from build123d import *

# Parameters (mm, degrees)
SKETCH1_R           = 4
BOSS_EXTRUDE1_DEPTH = 15
CUT_EXTRUDE1_REACH  = 24
SKETCH2_R           = 2
FILLET1_R           = 0.25


with BuildPart() as part:
    # Sketch1 → Boss-Extrude1 (new body, symmetric)
    with BuildSketch(Plane.XY):
        Polygon((17, -11), (-17, -11), (-17, 7), (-8.3, 7), (-4, 11), (4, 11), (8.3, 7), (17, 7), align=None)
        Circle(SKETCH1_R, mode=Mode.SUBTRACT)
    extrude(amount=BOSS_EXTRUDE1_DEPTH, both=True)

    # Sketch2 → Cut-Extrude1 (cut, up to next)
    with BuildSketch(Plane.XZ.offset(11), mode=Mode.PRIVATE) as cut_extrude1_sk1:
        with Locations((12, 9)):
            Circle(SKETCH2_R)
    cut_extrude1_tool1 = extrude(cut_extrude1_sk1.sketch, amount=-CUT_EXTRUDE1_REACH, mode=Mode.PRIVATE) & part.part
    add(cut_extrude1_tool1.solids().sort_by_distance((12, -11, 9))[0], mode=Mode.SUBTRACT)
    # Sketch2 → Cut-Extrude1 (cut, up to next)
    with BuildSketch(Plane.XZ.offset(11), mode=Mode.PRIVATE) as cut_extrude1_sk2:
        with Locations((-12, 9)):
            Circle(SKETCH2_R)
    cut_extrude1_tool2 = extrude(cut_extrude1_sk2.sketch, amount=-CUT_EXTRUDE1_REACH, mode=Mode.PRIVATE) & part.part
    add(cut_extrude1_tool2.solids().sort_by_distance((-12, -11, 9))[0], mode=Mode.SUBTRACT)
    # Sketch2 → Cut-Extrude1 (cut, up to next)
    with BuildSketch(Plane.XZ.offset(11), mode=Mode.PRIVATE) as cut_extrude1_sk3:
        with Locations((12, -9)):
            Circle(SKETCH2_R)
    cut_extrude1_tool3 = extrude(cut_extrude1_sk3.sketch, amount=-CUT_EXTRUDE1_REACH, mode=Mode.PRIVATE) & part.part
    add(cut_extrude1_tool3.solids().sort_by_distance((12, -11, -9))[0], mode=Mode.SUBTRACT)
    # Sketch2 → Cut-Extrude1 (cut, up to next)
    with BuildSketch(Plane.XZ.offset(11), mode=Mode.PRIVATE) as cut_extrude1_sk4:
        with Locations((-12, -9)):
            Circle(SKETCH2_R)
    cut_extrude1_tool4 = extrude(cut_extrude1_sk4.sketch, amount=-CUT_EXTRUDE1_REACH, mode=Mode.PRIVATE) & part.part
    add(cut_extrude1_tool4.solids().sort_by_distance((-12, -11, -9))[0], mode=Mode.SUBTRACT)

    # Fillet1
    fillet1_edges = [part.edges().sort_by_distance(p)[0] for p in [
        (0, 11, -15),
        (6.15, 9, -15),
        (12.65, 7, -15),
        (17, -2, -15),
        (6.15, 9, 15),
        (17, -11, 0),
        (-17, -11, 0),
        (-17, 7, 0),
        (-8.3, 7, 0),
        (-4, 11, 0),
        (4, 11, 0),
        (8.3, 7, 0),
        (17, 7, 0),
        (0, 11, 15),
        (-6.15, 9, 15),
        (-12.65, 7, 15),
        (-17, -2, 15),
        (0, -11, 15),
        (17, -2, 15),
        (0, -11, -15),
        (12.65, 7, 15),
        (-17, -2, -15),
        (-12.65, 7, -15),
        (-6.15, 9, -15),
    ]]
    fillet(fillet1_edges, radius=FILLET1_R)


solid = part.part
The listing builds one solid part. Answer for the finished solid, in the listing's coordinates (mm). A direction names the side the tool comes from. Round coordinates to 2 decimals unless told otherwise and drop trailing zeros. Order: outer loops, then holes, each group sorted by start corner. A loop starts at its lowest first (then second) coordinate and runs counter-clockwise, first axis right, second up. Notation, with made-up numbers: (6.5, 39) - (32.5, 39) arc R21 cw to (32.5, 52) - close; hole circle Ø1 at (62.5, 48.25). An arc over 180 degrees is marked (long way). Write item = value, one per line. Start each with the question number.
1) Section D-D, the plane x = 0 is taken. Write down the section's boundary in (y, z), plus the area to 3 significant figures.
2) Given pin 1 (4.5 mm diameter, centred on x = -12, z = 9, fed in from +Y); pin 2 (6.5 mm diameter, centred on x = -11, z = -3.5, fed in from +Y); pin 3 (2.5 mm diameter, centred on x = 12, z = 9, fed in from -Y), each flat-ended and moving along its own axis, determine where each tip first touches the part or whether it passes through.
3) For faces 4 (the flat face through (13, 7, 0)), 5 (the cylindrical face through (10.526, -2.126, -7.648)), 6 (the flat face through (-13, 7, 0)), determine the directions among +Z, -Z, +X, -X, +Y, -Y from which every point of the face is accessible in a straight line to the end or side of a thin tool.
4) Section B-B, the plane y = 0 is taken. Write down the section's boundary in (x, z), plus the area to 3 significant figures.
5) For a pull along Y with two mould halves and no side action, classify faces 1 (the flat face through (0, -5, -15)), 2 (the cylindrical face through (-6.07, 8.97, 14.93)), 3 (the cylindrical face through (-0.867, -3.905, -0.21)) as released by +Y, released by -Y, zero draft, split by the parting line, or undercut.
6) Section C-C, the plane x = -12 is taken. Write down the section's boundary in (y, z), plus the area to 3 significant figures.
7) Section A-A, the plane z = -9 is taken. Write down the section's boundary in (x, y).
8) Straight lines are drawn through the part: L1, parallel to Z at x = -12, y = -3.25; L2, parallel to Y at x = 0, z = -7.5; L3, parallel to X at y = 2.75, z = 7.5. For each, find the intervals that lie inside material, in ascending order.
Results list:
q1.outline = (-11, -14.75) arc R0.25 ccw to (-10.75, -15) - (-4, -15) - (-4, 15) - (-10.75, 15) arc R0.25 ccw to (-11, 14.75) - close; (4, -15) - (10.75, -15) arc R0.25 ccw to (11, -14.75) - (11, 14.75) arc R0.25 ccw to (10.75, 15) - (4, 15) - close
q1.area = 420 mm^2
q2.pin_1 = 7
q2.pin_2 = 7.51
q2.pin_3 = through
q3.face_4 = +Z, -Z, +X, +Y
q3.face_5 = +Y, -Y
q3.face_6 = +Z, -Z, -X, +Y
q4.outline = (-17, -14.75) arc R0.25 ccw to (-16.75, -15) - (-4, -15) - (-4, 15) - (-16.75, 15) arc R0.25 ccw to (-17, 14.75) - close; (4, -15) - (16.75, -15) arc R0.25 ccw to (17, -14.75) - (17, 14.75) arc R0.25 ccw to (16.75, 15) - (4, 15) - close; hole circle Ø4 at (-12, -9); hole circle Ø4 at (-12, 9); hole circle Ø4 at (12, -9); hole circle Ø4 at (12, 9)
q4.area = 730 mm^2
q5.face_1 = zero draft
q5.face_2 = released by +Y
q5.face_3 = undercut
q6.outline = (-11, -14.75) arc R0.25 ccw to (-10.75, -15) - (6.75, -15) arc R0.25 ccw to (7, -14.75) - (7, -11) - (-11, -11) - close; (-11, -7) - (7, -7) - (7, 7) - (-11, 7) - close; (-11, 11) - (7, 11) - (7, 14.75) arc R0.25 ccw to (6.75, 15) - (-10.75, 15) arc R0.25 ccw to (-11, 14.75) - close
q6.area = 396 mm^2
q7.outline = (-17, -10.75) arc R0.25 ccw to (-16.75, -11) - (-14, -11) - (-14, 7) - (-16.75, 7) arc R0.25 ccw to (-17, 6.75) - close; (-10, -11) - (10, -11) - (10, 7) - (8.4, 7) arc R0.25 cw to (8.23, 7.07) - (4.07, 10.93) arc R0.25 ccw to (3.9, 11) - (-3.9, 11) arc R0.25 ccw to (-4.07, 10.93) - (-8.23, 7.07) arc R0.25 cw to (-8.4, 7) - (-10, 7) - close; (14, -11) - (16.75, -11) arc R0.25 ccw to (17, -10.75) - (17, 6.75) arc R0.25 ccw to (16.75, 7) - (14, 7) - close; hole circle Ø8 at (0, 0)
q8.L1 = -15 to -11, -7 to 7, 11 to 15
q8.L2 = -11 to -4, 4 to 11
q8.L3 = -17 to -13.32, -10.68 to -2.9, 2.9 to 10.68, 13.32 to 17
